from build123d import *

# Parameters (mm, degrees)
SKETCH1_W           = 450
SKETCH1_H           = 300
BOSS_EXTRUDE1_DEPTH = 75
SHELL1_T            = -10
CUT_EXTRUDE1_DEPTH  = 451
CUT_EXTRUDE2_DEPTH  = 301
SKETCH4_R           = 7.5
SKETCH4_R_2         = 5
BOSS_EXTRUDE2_DEPTH = 15
BOSS_EXTRUDE2_TAPER = 2
SKETCH5_R           = 5.523811542
CUT_EXTRUDE3_DEPTH  = 15
BOSS_EXTRUDE3_DEPTH = 15
SKETCH8_W           = 90
SKETCH8_H           = 90
CUT_EXTRUDE5_DEPTH  = 5
SKETCH9_R           = 5
CUT_EXTRUDE6_DEPTH  = 65
SKETCH11_W          = 280
SKETCH11_H          = 15
CUT_EXTRUDE8_DEPTH  = 271


with BuildPart() as part:
    # Sketch1 → Boss-Extrude1 (new body)
    with BuildSketch(Plane(origin=(0, 0, 0), x_dir=(1, 0, 0), z_dir=(0, 1, 0))):
        Rectangle(SKETCH1_W, SKETCH1_H)
    extrude(amount=BOSS_EXTRUDE1_DEPTH)

    # Shell1
    shell1_openings = [part.faces().sort_by_distance(p)[0] for p in [
        (0, 0, 0),
    ]]
    offset(amount=SHELL1_T, openings=shell1_openings, kind=Kind.INTERSECTION)

    # Sketch2 → Cut-Extrude1 (cut, through all)
    with BuildSketch(Plane(origin=(225, 0, 0), x_dir=(0, 0, -1), z_dir=(1, 0, 0))):
        with BuildLine():
            Line((-102.5, 25), (102.5, 25))
            ThreePointArc((102.5, 25), (109.571067812, 22.071067812), (112.5, 15))
            Line((112.5, 15), (112.5, -15))
            ThreePointArc((112.5, -15), (109.571067812, -22.071067812), (102.5, -25))
            Line((102.5, -25), (-102.5, -25))
            ThreePointArc((-102.5, -25), (-109.571067812, -22.071067812), (-112.5, -15))
            Line((-112.5, -15), (-112.5, 15))
            ThreePointArc((-112.5, 15), (-109.571067812, 22.071067812), (-102.5, 25))
        make_face()
    extrude(amount=-CUT_EXTRUDE1_DEPTH, mode=Mode.SUBTRACT)

    # Sketch3 → Cut-Extrude2 (cut, through all)
    with BuildSketch(Plane.XY.offset(150)):
        with BuildLine():
            Line((-190, -25), (190, -25))
            ThreePointArc((190, -25), (197.071067812, -22.071067812), (200, -15))
            Line((200, -15), (200, 15))
            ThreePointArc((200, 15), (197.071067812, 22.071067812), (190, 25))
            Line((190, 25), (-190, 25))
            ThreePointArc((-190, 25), (-197.071067812, 22.071067812), (-200, 15))
            Line((-200, 15), (-200, -15))
            ThreePointArc((-200, -15), (-197.071067812, -22.071067812), (-190, -25))
        make_face()
    extrude(amount=-CUT_EXTRUDE2_DEPTH, mode=Mode.SUBTRACT)

    # Sketch4 → Boss-Extrude2 (add)
    with BuildSketch(Plane(origin=(0, 75, 0), x_dir=(1, 0, 0), z_dir=(0, 1, 0))):
        with Locations((-200, 125)):
            Circle(SKETCH4_R)
        with Locations((-200, 125)):
            Circle(SKETCH4_R_2, mode=Mode.SUBTRACT)
    extrude(amount=BOSS_EXTRUDE2_DEPTH, taper=BOSS_EXTRUDE2_TAPER)

    # Sketch5 → Cut-Extrude3 (cut)
    with BuildSketch(Plane(origin=(0, 75, 0), x_dir=(1, 0, 0), z_dir=(0, 1, 0))):
        with Locations((-200, 125)):
            Circle(SKETCH5_R)
    extrude(amount=-CUT_EXTRUDE3_DEPTH, mode=Mode.SUBTRACT)

    # Sketch6 → Boss-Extrude3 (add)
    with BuildSketch(Plane(origin=(0, 75, 0), x_dir=(1, 0, 0), z_dir=(0, 1, 0))):
        with BuildLine():
            Line((-105, 120), (175, 120))
            Line((175, 120), (175, 37.5))
            ThreePointArc((175, 37.5), (137.5, 0), (175, -37.5))
            Line((175, -37.5), (175, -120))
            Line((175, -120), (-105, -120))
            Line((-105, -120), (-105, 120))
        make_face()
        Polygon((135, 80), (0, 80), (0, 105), (-65, 105), (-65, 25), (0, 25), (0, 50), (135, 50), align=None, mode=Mode.SUBTRACT)
        Polygon((135, -50), (135, -80), (0, -80), (0, -105), (-65, -105), (-65, -25), (0, -25), (0, -50), align=None, mode=Mode.SUBTRACT)
    extrude(amount=BOSS_EXTRUDE3_DEPTH)

    # Sketch8 → Cut-Extrude5 (cut)
    with BuildSketch(Plane(origin=(0, 75, 0), x_dir=(1, 0, 0), z_dir=(0, 1, 0))):
        with Locations((-160, 0)):
            Rectangle(SKETCH8_W, SKETCH8_H)
    extrude(amount=-CUT_EXTRUDE5_DEPTH, mode=Mode.SUBTRACT)

    # Sketch9 → Cut-Extrude6 (cut)
    with BuildSketch(Plane(origin=(0, 70, 0), x_dir=(1, 0, 0), z_dir=(0, 1, 0))):
        with Locations((-195, 35)):
            Circle(SKETCH9_R)
        with Locations((-125, 35)):
            Circle(SKETCH9_R)
        with Locations((-125, -35)):
            Circle(SKETCH9_R)
        with Locations((-195, -35)):
            Circle(SKETCH9_R)
    extrude(amount=-CUT_EXTRUDE6_DEPTH, mode=Mode.SUBTRACT)

    # Sketch11 → Cut-Extrude8 (cut, through all)
    with BuildSketch(Plane.XY.offset(120)):
        with Locations((35, 82.5)):
            Rectangle(SKETCH11_W, SKETCH11_H)
    extrude(amount=-CUT_EXTRUDE8_DEPTH, mode=Mode.SUBTRACT)


solid = part.part
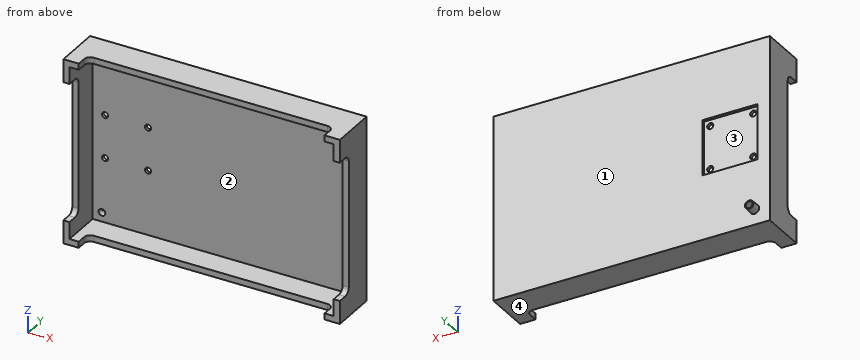
The listing builds one solid part. Answer for the finished solid, in the listing's coordinates (mm). Face numbers are marked on the shaded views. Round coordinates to 2 decimals unless told otherwise and drop trailing zeros. Write each loop counter-clockwise with the first axis right and the second up, starting at its lowest first coordinate (ties: lowest second). Pieces come first, ordered by that corner, then holes. Notation, with made-up numbers: (34.25, 34.5) - (53.25, 34.5) arc R18 cw to (53.25, 49.5) - close; hole circle Ø6 at (58, 67). An arc over 180 degrees is marked (long way). Use one line per item in the form item = value. Start each with the question number.
Item 1: Determine the mould class of the marked faces 1, 2, 3 and 4 for opening direction Z: +Z half, -Z half, draft (parallel to the pull), parting line (faces both ways), or undercut.
Item 2: Flat-ended cylindrical pins translate along their axes: pin 1 Ø11 at (x, z) = (-222, 48) entering from -Y; pin 2 Ø13 at (x, z) = (-125, -35) entering from +Y; pin 3 Ø5 at (x, z) = (-109, -34) entering from +Y. Find the tip coordinate at first contact, or state that the pin passes through.
Item 3: A cutting plane is placed at A-A (z = 35). Write down the section's boundary in (x, y).
Item 4: A cutting plane is placed at C-C (y = 49). Write down the section's boundary in (x, z), plus the area to 3 significant figures.
Item 5: Find the intervals of material crossed by line 1 (X direction, y = 66.6, z = -35); line 2 (Z direction, x = -125, y = 68); line 3 (X direction, y = 42.5, z = -63.5), in increasing order. Write a range as [from, to].
Item 6: A cutting plane is placed at B-B (x = -144.5). Write down the section's boundary in (y, z), plus the area to 3 significant figures.
Item 7: A cutting plane is placed at D-D (z = 88.5). Write down the section's boundary in (x, y), plus the area to 3 significant figures.
The answers:
q1.face_1 = draft
q1.face_2 = undercut
q1.face_3 = undercut
q1.face_4 = -Z half
q2.pin_1 = 25
q2.pin_2 = 70
q2.pin_3 = 75
q3.outline = (-225, 25) - (-215, 25) - (-215, 65) - (-200, 65) - (-200, 70) - (-205, 70) - (-205, 75) - (-225, 75) - close; (-190, 65) - (-130, 65) - (-130, 70) - (-190, 70) - close; (-120, 65) - (215, 65) - (215, 25) - (225, 25) - (225, 75) - (-115, 75) - (-115, 70) - (-120, 70) - close
q4.outline = (-225, -150) - (225, -150) - (225, 150) - (-225, 150) - close; hole (-215, -140) - (215, -140) - (215, 140) - (-215, 140) - close
q4.area = 14,600 mm^2
q5.line_1 = [-225, -200], [-190, -130], [-120, 225]
q5.line_2 = [-150, -40], [-30, 30], [40, 150]
q5.line_3 = [-225, -215], [215, 225]
q6.outline = (25, -150) - (75, -150) - (75, -45) - (70, -45) - (70, 45) - (75, 45) - (75, 150) - (25, 150) - (25, 140) - (65, 140) - (65, -140) - (25, -140) - close
q6.area = 3,350 mm^2
q7.outline = (-225, 25) - (-215, 25) - (-215, 65) - (215, 65) - (215, 25) - (225, 25) - (225, 75) - (-225, 75) - close
q7.area = 5,300 mm^2
